Read the model definition and answer for the solid it produces. Units are mm, in the model's axes. Give positions to 0.01 mm unless a question says otherwise; leave off trailing zeros. Order: outer loops, then holes, each group sorted by start corner. A loop starts at its lowest first (then second) coordinate and runs counter-clockwise, first axis right, second up. Notation, with made-up numbers: M -40,33 L 6,33 A15 cw 6,58 Z; hole C 45,-35.5 d10. An arc over 180 degrees is marked long. Write item = value, one per line. Start each with the question number.
from build123d import *

# Parameters (mm, degrees)
SKETCH1_W           = 101.6
SKETCH1_H           = 50.8
BOSS_EXTRUDE1_DEPTH = 6.35
CUT_EXTRUDE2_REACH  = 59.15
SKETCH3_R           = 3.429


with BuildPart() as part:
    # Sketch1 → Boss-Extrude1 (new body)
    with BuildSketch(Plane(origin=(0, 0, 0), x_dir=(1, 0, 0), z_dir=(0, 1, 0))):
        Rectangle(SKETCH1_W, SKETCH1_H)
    extrude(amount=BOSS_EXTRUDE1_DEPTH)

    # Sketch3 → Cut-Extrude2 (cut, up to next)
    with BuildSketch(Plane.XZ, mode=Mode.PRIVATE) as cut_extrude2_sk1:
        with Locations(Location((-38.1, 12.7, 0), (0, 0, 270))):
            Circle(SKETCH3_R)
    cut_extrude2_tool1 = extrude(cut_extrude2_sk1.sketch, amount=-CUT_EXTRUDE2_REACH, mode=Mode.PRIVATE) & part.part
    # Sketch3 → Cut-Extrude2 (cut, up to next)
    with BuildSketch(Plane.XZ, mode=Mode.PRIVATE) as cut_extrude2_sk2:
        with Locations(Location((-38.1, -12.7, 0), (0, 0, 90))):
            Circle(SKETCH3_R)
    cut_extrude2_tool2 = extrude(cut_extrude2_sk2.sketch, amount=-CUT_EXTRUDE2_REACH, mode=Mode.PRIVATE) & part.part
    # Sketch3 → Cut-Extrude2 (cut, up to next)
    with BuildSketch(Plane.XZ, mode=Mode.PRIVATE) as cut_extrude2_sk3:
        with Locations(Location((38.1, 12.7, 0), (0, 0, 90))):
            Circle(SKETCH3_R)
    cut_extrude2_tool3 = extrude(cut_extrude2_sk3.sketch, amount=-CUT_EXTRUDE2_REACH, mode=Mode.PRIVATE) & part.part
    # Sketch3 → Cut-Extrude2 (cut, up to next)
    with BuildSketch(Plane.XZ, mode=Mode.PRIVATE) as cut_extrude2_sk4:
        with Locations(Location((38.1, -12.7, 0), (0, 0, 270))):
            Circle(SKETCH3_R)
    cut_extrude2_tool4 = extrude(cut_extrude2_sk4.sketch, amount=-CUT_EXTRUDE2_REACH, mode=Mode.PRIVATE) & part.part
    add(cut_extrude2_tool1.solids().sort_by_distance((-38.1, 0, 12.7))[0], mode=Mode.SUBTRACT)
    add(cut_extrude2_tool2.solids().sort_by_distance((-38.1, 0, -12.7))[0], mode=Mode.SUBTRACT)
    add(cut_extrude2_tool3.solids().sort_by_distance((38.1, 0, 12.7))[0], mode=Mode.SUBTRACT)
    add(cut_extrude2_tool4.solids().sort_by_distance((38.1, 0, -12.7))[0], mode=Mode.SUBTRACT)


solid = part.part
1) Find section C-C on y = 2.75. Determine the outline of the cut face in (x, z), plus the area to 3 significant figures.
2) Find section B-B on z = 12.7. Determine the outline of the cut face in (x, y), plus the area to 3 significant figures.
3) For a pull along Z with two mould halves and no side action, classify faces 1 (the face through (-1, 3, -25.4)), 2 (the face through (-1, 6.35, 0)), 3 (the face through (38.251, 3.131, -9.274)), 4 (the face through (-39.13, 3.13, -9.43)) as pulls with the +Z half, pulls with the -Z half, needs draft (parallel to the pull), parting line crosses it, or undercut.
4) Find the intervals of material crossed by probe 1 along Z at (x, y) = (38, 1.5); probe 2 along X at (y, z) = (1.5, -12.7); probe 3 along X at (y, z) = (2.5, 13.5), in increasing order. Write a range as [from, to].
5) Find section A-A on x = 38.1. Determine the outline of the cut face in (y, z), plus the area to 3 significant figures.
Numbers:
q1.outline = M -50.8,-25.4 L 50.8,-25.4 L 50.8,25.4 L -50.8,25.4 Z; hole C -38.1,-12.7 d6.86; hole C -38.1,12.7 d6.86; hole C 38.1,-12.7 d6.86; hole C 38.1,12.7 d6.86
q1.area = 5,010 mm2
q2.outline = M -50.8,0 L -41.53,0 L -41.53,6.35 L -50.8,6.35 Z; M -34.67,0 L 34.67,0 L 34.67,6.35 L -34.67,6.35 Z; M 41.53,0 L 50.8,0 L 50.8,6.35 L 41.53,6.35 Z
q2.area = 558 mm2
q3.face_1 = pulls with the -Z half
q3.face_2 = needs draft
q3.face_3 = undercut
q3.face_4 = undercut
q4.probe_1 = [-25.4, -16.13], [-9.27, 9.27], [16.13, 25.4]
q4.probe_2 = [-50.8, -41.53], [-34.67, 34.67], [41.53, 50.8]
q4.probe_3 = [-50.8, -41.43], [-34.77, 34.77], [41.43, 50.8]
q5.outline = M 0,-25.4 L 6.35,-25.4 L 6.35,-16.13 L 0,-16.13 Z; M 0,-9.27 L 6.35,-9.27 L 6.35,9.27 L 0,9.27 Z; M 0,16.13 L 6.35,16.13 L 6.35,25.4 L 0,25.4 Z
q5.area = 235 mm2
